Work out the finished part from the listing and answer in its coordinate system (mm). A direction names the side the tool comes from. Round coordinates to 2 decimals unless told otherwise and drop trailing zeros. Loops run counter-clockwise (first coordinate to the right, second up) from the corner with the lowest first, then second, coordinate; pieces in that order, holes last. Notation, with made-up numbers: (61.5, -6.5) - (101.5, -6.5) arc R21 ccw to (101.5, 28.5) - close; hole circle Ø9 at (25, 29.5). An arc over 180 degrees is marked (long way). Return JSON: item names as keys, results as strings.
Autodesk Inventor part; units mm, degrees
ref_plane "YZ Plane" through (0, 0, 0) normal (1, 0, 0) x (0, 1, 0)
ref_plane "XZ Plane" through (0, 0, 0) normal (0, 1, 0) x (-1, 0, 0)
sketch "Skizze1" plane through (0, 0, 0) normal (0, 0, 1) x (1, 0, 0)
  line L0 (0, 0) -> (0, 22)
  line L1 (0, 22) -> (107, 22)
  line L2 (107, 22) -> (107, 30)
  line L3 (107, 30) -> (131.65, 30)
  line L4 (131.65, 30) -> (131.65, 36.5)
  line L5 (131.65, 36.5) -> (153.65, 36.5)
  line L6 (153.65, 36.5) -> (153.65, 30)
  line L7 (153.65, 30) -> (178.3, 30)
  line L8 (178.3, 30) -> (178.3, 0)
  line L9 (178.3, 0) -> (0, 0)
  line L10 (-35.66, 0) -> (213.96, 0)
revolve "Umdrehung1" add sketch "Skizze1" angle 360 about axis through (-10, 0, 0) along (1, 0, 0)
ref_plane "Arbeitsebene1" through (0, 0, 22) normal (0, 0, 1) x (1, 0, 0)
sketch "Skizze2" plane through (0, 0, 22) normal (0, 0, 1) x (1, 0, 0)
  line L0 (8.5, 0) -> (98.5, 0) construction
  line L1 (14.5, -6) -> (92.5, -6)
  line L2 (92.5, 6) -> (14.5, 6)
  arc A0 (14.5, 6) -> (14.5, -6) centre (14.5, 0) ccw
  arc A1 (92.5, -6) -> (92.5, 6) centre (92.5, 0) ccw
  point P0 (53.5, 0)
extrude "Extrusion1" cut sketch "Skizze2" against normal blind 5
sketch "Skizze3" plane through (0, 0, 0) normal (0, 0, 1) x (1, 0, 0)
  line L0 (107, 24) -> (107.2, 23.2536)
  line L1 (105.6196, 21.7) -> (104.5, 22)
  line L2 (104.5, 22) -> (104.5, 24)
  line L3 (104.5, 24) -> (107, 24)
  arc A0 (105.6196, 21.7) -> (107.2, 23.2536) centre (106.1294, 22.762) ccw
  line L4 (-35.66, 0) -> (213.96, 0)
revolve "Umdrehung2" cut sketch "Skizze3" angle 360 about axis through (-10, 0, 0) along (1, 0, 0)
sketch "Skizze4" plane through (0, 0, 0) normal (0, 0, 1) x (1, 0, 0)
  line L0 (111.5, 28.5) -> (113.65, 28.5)
  line L1 (113.65, 28.5) -> (113.65, 30)
  line L2 (113.65, 30) -> (111.5, 30)
  line L3 (111.5, 30) -> (111.5, 28.5)
  line L4 (-35.66, 0) -> (213.96, 0)
revolve "Umdrehung3" cut sketch "Skizze4" angle 360 about axis through (-10, 0, 0) along (1, 0, 0)
sketch "Skizze5" plane through (0, 0, 0) normal (0, 0, 1) x (1, 0, 0)
  line L0 (131.65, 32) -> (131.85, 31.2536)
  line L1 (130.2696, 29.7) -> (129.15, 30)
  line L2 (129.15, 30) -> (129.15, 32)
  line L3 (129.15, 32) -> (131.65, 32)
  arc A0 (130.2696, 29.7) -> (131.85, 31.2536) centre (130.7794, 30.762) ccw
  line L4 (-35.66, 0) -> (213.96, 0)
revolve "Umdrehung4" cut sketch "Skizze5" angle 360 about axis through (-10, 0, 0) along (1, 0, 0)
sketch "Skizze6" plane through (0, 0, 0) normal (0, 0, 1) x (1, 0, 0)
  line L0 (173.8, 28.5) -> (171.65, 28.5)
  line L1 (171.65, 28.5) -> (171.65, 30)
  line L2 (171.65, 30) -> (173.8, 30)
  line L3 (173.8, 30) -> (173.8, 28.5)
  line L4 (-35.66, 0) -> (213.96, 0)
revolve "Umdrehung5" cut sketch "Skizze6" angle 360 about axis through (-10, 0, 0) along (1, 0, 0)
sketch "Skizze7" plane through (0, 0, 0) normal (0, 0, 1) x (1, 0, 0)
  line L0 (153.65, 32) -> (153.45, 31.2536)
  line L1 (155.0304, 29.7) -> (156.15, 30)
  line L2 (156.15, 30) -> (156.15, 32)
  line L3 (156.15, 32) -> (153.65, 32)
  arc A0 (153.45, 31.2536) -> (155.0304, 29.7) centre (154.5206, 30.762) ccw
  line L4 (-35.66, 0) -> (213.96, 0)
revolve "Umdrehung6" cut sketch "Skizze7" angle 360 about axis through (-10, 0, 0) along (1, 0, 0)
1) Find the intervals of material crossed by L1, parallel to X at y = -30, z = -19; L2, parallel to X at y = 0, z = -26.5; L3, parallel to Z at x = 46, y = 0.5, in increasing order.
Verdict:
{"L1": "x = 131.65 to 153.65", "L2": "x = 107 to 178.3", "L3": "z = -21.99 to 17"}
2) A tool of negligible diameter and unlimited length cuts with its end or side. For faces 4 (the cylindrical face through (98.5, -0.1, 19.5)), 5 (the cylindrical face through (52.982, -4.769, -21.477)), 6 (the flat face through (0, 0, 0)), 7 (the flat face through (173.8, 11, -27)), 8 (the flat face through (153.65, -0.2, -32.3)), from which of +Z, -Z, +X, -X, +Y, -Y can it reach the whole face along a straight path? Write none if from no direction.
Verdict:
{"face 4": "+Z", "face 5": "-X", "face 6": "+Z, -Z, -X, +Y, -Y", "face 7": "none", "face 8": "+X"}
3) Flat-ended cylindrical pins translate along their axes: pin 1 (3 mm diameter, centred on x = 49.5, y = -12, fed in from -Z); pin 2 (5 mm diameter, centred on y = 21, z = -17, fed in from -X); pin 3 (8 mm diameter, centred on x = 48.5, z = 24, fed in from +Y). Find the tip coordinate at first contact, or state that the pin passes through.
Verdict:
{"pin 1": "stops at z = -19.33", "pin 2": "stops at x = 107", "pin 3": "stops at y = 9.17"}
4) Section B-B (x = 51.5) is taken. Give the vertices of the cut face in (y, z).
Verdict:
{"outline": "(-6, 17) - (-6, 21.17) arc R22 ccw (long way) to (6, 21.17) - (6, 17) - close"}
5) Section A-A (x = 163) is taken. Give the vertices of the cut face in (y, z), and give its area (3 significant figures).
Verdict:
{"outline": "circle Ø60 at (0, 0)", "area": "2,830 mm2"}
6) Determine the mould class of faces 1 (the cylindrical face through (172.71, 26.327, 10.916)), 2 (the flat face through (131.65, -0.2, -32.3)), 3 (the flat face through (53, 0, 17)) for opening direction Y: pulls with the +Y half, pulls with the -Y half, needs draft (parallel to the pull), parting line crosses it, or undercut.
Verdict:
{"face 1": "parting line crosses it", "face 2": "needs draft", "face 3": "undercut"}
